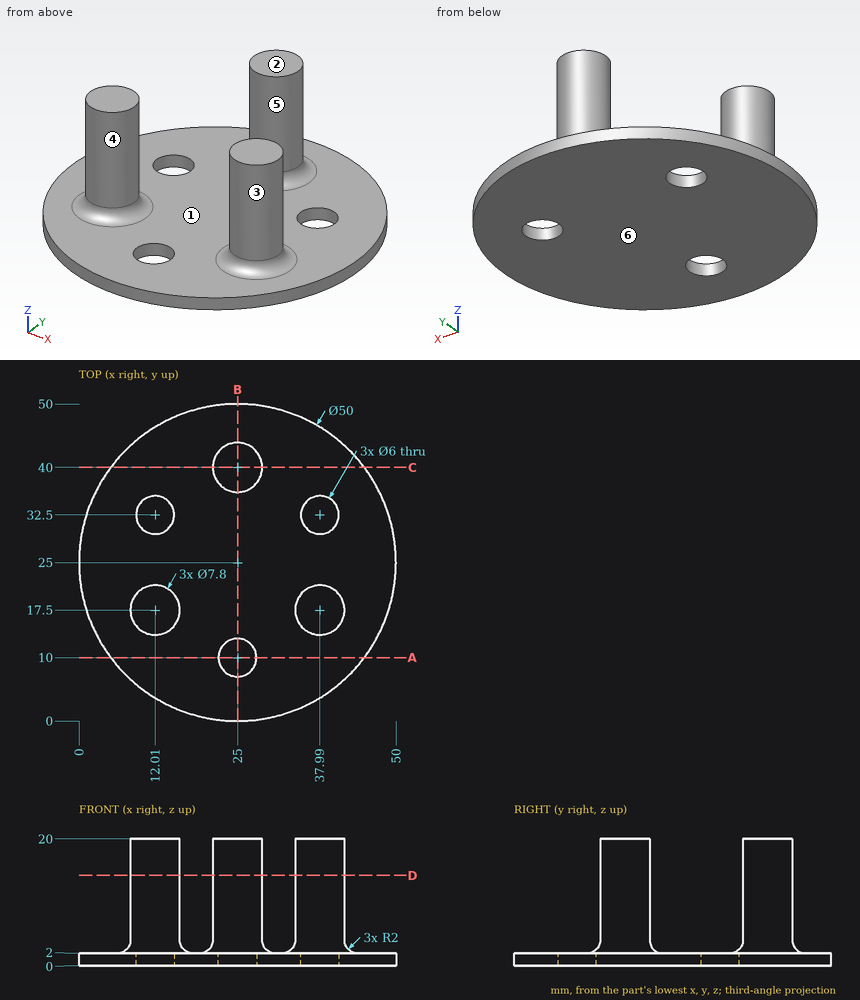
Geometry: see drawing. Coordinates: mm, zero at the bounding-box minimum. A direction names the side the tool comes from. Coordinates: 2 decimals unless noted, no trailing zeros. Loops run counter-clockwise (first coordinate to the right, second up) from the corner with the lowest first, then second, coordinate; pieces in that order, holes last.
Q1. Cut plane C-C (y = 40). Output: boundary loops of the cut face in (x, z).
Q2. Cut plane B-B (x = 25). Output: boundary loops of the cut face in (y, z).
Q3. Material intervals for line 1 (Y direction, x = 25, z = 0.95); line 2 (Z direction, x = 10.5, y = 42); line 3 (X direction, y = 21, z = 17.5), sorted ascending.
Q4. Contact query for flat-ended pins moving along their axis: pin 1 (2 mm diameter, centred on y = 38.5, z = 7, fed in from -X); pin 2 (2 mm diameter, centred on y = 16, z = 6, fed in from -X); pin 3 (1 mm diameter, centred on x = 36.5, z = 17.5, fed in from +Y). Output: stop coordinate, or through.
Q5. Cut plane A-A (y = 10). Output: boundary loops of the cut face in (x, z).
Q6. Set-up query: the marked faces 1 and 2. Return all of +Z, -Z, +X, -X, +Y, -Y with unobstructed straight access to the full face (end or side cutting, diameter ignored); none if empty.
Q7. Draft query along X for the marked faces 3, 4, 5 and 6. Return one class per face: +X half, -X half, draft (parallel to the pull), parting line (faces both ways), or undercut.
Q8. Cut plane D-D (z = 14.25). Output: boundary loops of the cut face in (x, y).
Working result:
1. outline: (5, 0) - (45, 0) - (45, 2) - (30.9, 2) arc R2 cw to (28.9, 4) - (28.9, 20) - (21.1, 20) - (21.1, 4) arc R2 cw to (19.1, 2) - (5, 2) - close
2. outline: (0, 0) - (7, 0) - (7, 2) - (0, 2) - close; (13, 0) - (50, 0) - (50, 2) - (45.9, 2) arc R2 cw to (43.9, 4) - (43.9, 20) - (36.1, 20) - (36.1, 4) arc R2 cw to (34.1, 2) - (13, 2) - close
3. line 1: y = 0 to 7, 13 to 50
3. line 2: z = 0 to 2
3. line 3: x = 10.29 to 13.73, 36.27 to 39.71
4. pin 1: stops at x = 21.13
4. pin 2: stops at x = 8.14
4. pin 3: stops at y = 21.27
5. outline: (5, 0) - (22, 0) - (22, 2) - (5, 2) - close; (28, 0) - (45, 0) - (45, 2) - (28, 2) - close
6. face 1: +Z
6. face 2: +Z, +X, -X, +Y, -Y
7. face 3: undercut
7. face 4: undercut
7. face 5: parting line
7. face 6: draft
8. outline: circle Ø7.8 at (12.01, 17.5); circle Ø7.8 at (25, 40); circle Ø7.8 at (37.99, 17.5)
